Build history of the part. All positions in model axes, mm. A direction names the side the tool comes from. Round coordinates to 2 decimals unless told otherwise and drop trailing zeros. Write each loop counter-clockwise with the first axis right and the second up, starting at its lowest first coordinate (ties: lowest second). Pieces come first, ordered by that corner, then holes.
Item 1: Wall check: probe 1 along Y at (x, z) = (12, -16.25); probe 2 along Y at (x, z) = (107.5, -17.25); probe 3 along X at (y, z) = (-111, -0.8). Give the ranges that are in metal, low to high.
Item 2: Band-saw the part on A-A, the plane z = -16.5. Write the cut outline in (x, y) (3 decimals).
Item 3: Drop flat-ended pins along their axis: pin 1 Ø4 at (x, z) = (-153, -5.5) entering from +Y; pin 2 Ø7 at (x, y) = (-214.44, 57.46) entering from -Z; pin 3 Ø7 at (x, y) = (-111, 192.26) entering from +Z; pin 4 Ø1.5 at (x, z) = (105.5, -2.5) entering from +Y. Give the stop position or say it passes through.
Item 4: Mould opens along Y. For faces 3 (the flat face through (-119, 186, 0)), 4 (the cylindrical face through (-160.25, 146.95, -11.43)), 5 (the cylindrical face through (206.336, 64.978, -11.619)) say: +Y half, -Y half, draft (parallel to the pull), parting line (faces both ways), or undercut.
Item 5: 3-axis set-ups, long thin cutter, end or side, ignore diameter. For faces 1 (the flat face through (-119, 186, -1.1)), 2 (the cylindrical face through (-49.28, -221.92, -0.54)): which of +Z, -Z, +X, -X, +Y, -Y reach the whole face in a straight line?
```python
from build123d import *

# Parameters (mm, degrees)
M4_CLEARANCE_HOLE1_D = 4.5
CIRPATTERN1_COUNT    = 24
SKETCH6_R            = 2.25
SKETCH6_R_2          = 2
BOSS_EXTRUDE1_DEPTH  = 1.1


with BuildPart() as part:
    # Sweep1: sweep along a path in Sketch1
    with BuildLine(Plane.XY) as sweep1_path:
        CenterArc((0, 0), 216.325, 0, 360)
    # Sketch2 → Sweep1 (sweep)
    with BuildSketch(Plane(origin=(0, 0, 0), x_dir=(0, 0, -1), z_dir=(1, 0, 0))):
        with BuildLine():
            Line((0, 227.325), (0, 219.325))
            ThreePointArc((0, 219.325), (0.878679656, 217.203679656), (3, 216.325))
            Line((3, 216.325), (20, 216.325))
            Line((20, 216.325), (20, 217.425))
            Line((20, 217.425), (3.1, 217.425))
            ThreePointArc((3.1, 217.425), (1.685786438, 218.010786438), (1.1, 219.425))
            Line((1.1, 219.425), (1.1, 227.325))
            Line((1.1, 227.325), (0, 227.325))
        make_face()
    sweep(path=sweep1_path.line)

    # M4 Clearance Hole1 (through all)
    with Locations(Plane.XY):
        with Locations((0, 222)):
            m4_clearance_hole1 = Hole(M4_CLEARANCE_HOLE1_D / 2)

    # CirPattern1: M4 Clearance Hole1 ×24 about axis
    cirpattern1_axis = Axis((0, 0, 0), (0, 0, 1))
    for i in range(1, CIRPATTERN1_COUNT):
        add(m4_clearance_hole1.rotate(cirpattern1_axis, i * 360 / CIRPATTERN1_COUNT), mode=Mode.SUBTRACT)

    # Sketch6 → Boss-Extrude1 (add)
    with BuildSketch(Plane.XY):
        with Locations((-222, 0)):
            Circle(SKETCH6_R)
        with Locations((-222, 0)):
            Circle(SKETCH6_R_2, mode=Mode.SUBTRACT)
        with Locations((222, 0)):
            Circle(SKETCH6_R)
        with Locations((222, 0)):
            Circle(SKETCH6_R_2, mode=Mode.SUBTRACT)
    extrude(amount=-BOSS_EXTRUDE1_DEPTH)


solid = part.part
```
Results:
1. probe 1: y = -217.09 to -215.99, 215.99 to 217.09
1. probe 2: y = -188.99 to -187.72, 187.72 to 188.99
1. probe 3: x = -198.38 to -194.51, -190.01 to -186.79, 186.79 to 190.01, 194.51 to 198.38
2. outline: circle Ø434.85 at (0, 0); hole circle Ø432.65 at (0, 0)
3. pin 1: stops at y = 156.44
3. pin 2: stops at z = -1.32
3. pin 3: stops at z = 0
3. pin 4: stops at y = 190.82
4. face 3: draft
4. face 4: parting line
4. face 5: undercut
5. face 1: -Z
5. face 2: +Z, -Z
